Study the drawing (mm; zero at the part's minimum x, y, z) and answer. A direction names the side the tool comes from. Give positions to 0.01 mm unless a question says otherwise; leave off trailing zeros. Write each loop counter-clockwise with the first axis right and the second up, starting at its lowest first coordinate (ties: lowest second). Pieces come first, ordered by that corner, then holes. Notation, with made-up numbers: (-19, 59.25) -> (2, 59.25) arc R28 ccw to (2, 78.25) -> close; hole circle Ø1 at (74, -37). An arc over 180 degrees is marked (long way). Use CSV: the item, a comma, the result in double quotes. Start each with the question number.
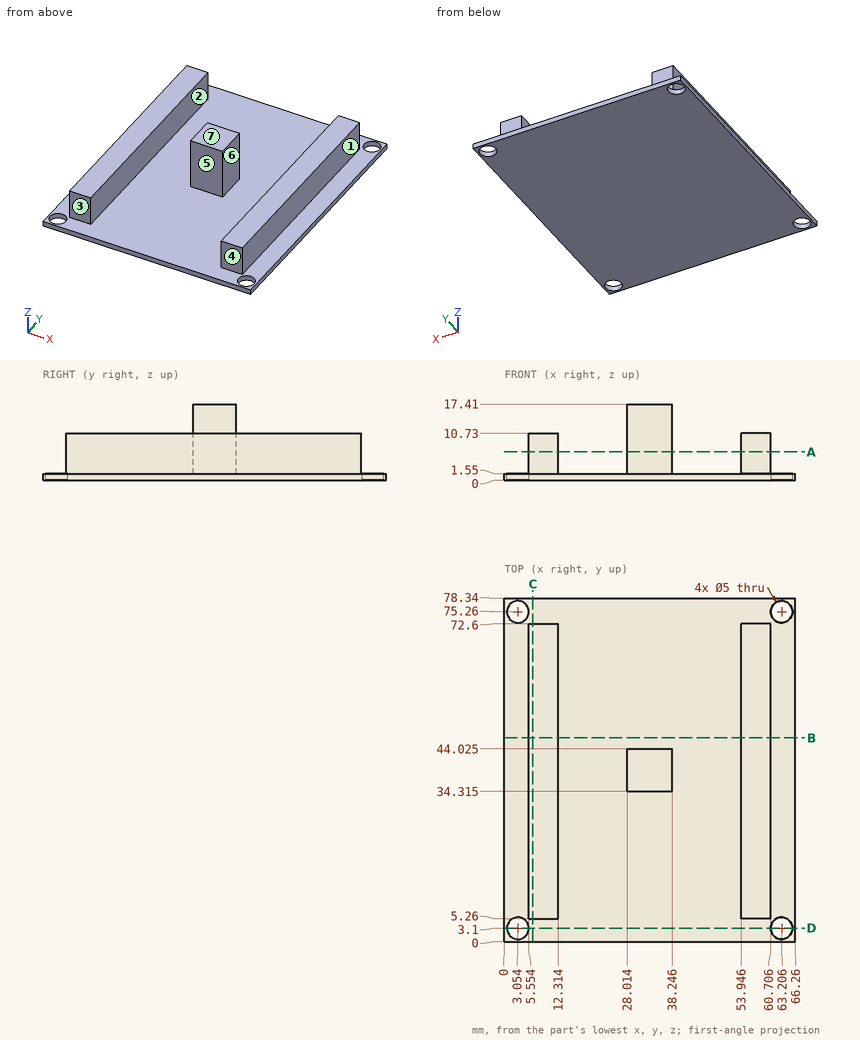
Q1. Straight lines are drawn through the part: L1, parallel to X at y = 41, z = 2; L2, parallel to X at y = 56, z = 5.25; L3, parallel to Z at x = 46.5, y = 47.5. For each, find the intervals that lie inside material, in ascending order.
Q2. Section A-A on z = 6.5 is taken. Give the vertices of the cut face in (x, y) (1 decimal).
Q3. Flat-ended cylindrical pins translate along their axes: pin 1 Ø6.5 at (x, y) = (3.05, 3.1) entering from +Z; pin 2 Ø8 at (y, z) = (40.5, 10.5) entering from +X; pin 3 Ø4.5 at (y, z) = (27.5, 6) entering from -X. Find the tip coordinate at first contact, or state that the pin passes through.
Q4. Section C-C on x = 6.5 is taken. Give the vertices of the cut face in (y, z).
Q5. Section D-D on y = 3.1 is taken. Give the vertices of the cut face in (x, z).
Q6. Section B-B on y = 46.5 is taken. Give the vertices of the cut face in (x, z), then the cut area to 3 significant figures.
Q7. For the marked faces 4, 5, 6 and 7, determine the directions among +Z, -Z, +X, -X, +Y, -Y from which every point of the face is accessible in a straight line to the end or side of a thin tool.
Q8. The mould has two halves that part along X. Classify the marked faces 1, 2 and 3: +X half, -X half, draft (parallel to the pull), parting line (faces both ways), or undercut.
Output:
1,L1,"5.55 to 12.31, 28.01 to 38.25, 53.95 to 60.71"
1,L2,"5.55 to 12.31, 53.95 to 60.71"
1,L3,"0 to 1.55"
2,outline,"(5.6, 5.3) -> (12.3, 5.3) -> (12.3, 72.6) -> (5.6, 72.6) -> close; (28, 34.3) -> (38.2, 34.3) -> (38.2, 44) -> (28, 44) -> close; (53.9, 5.3) -> (60.7, 5.3) -> (60.7, 72.6) -> (53.9, 72.6) -> close"
3,pin 1,"z = 1.55"
3,pin 2,"x = 60.71"
3,pin 3,"x = 5.55"
4,outline,"(0, 0) -> (78.34, 0) -> (78.34, 1.55) -> (72.6, 1.55) -> (72.6, 10.73) -> (5.26, 10.73) -> (5.26, 1.55) -> (0, 1.55) -> close"
5,outline,"(0, 0) -> (0.55, 0) -> (0.55, 1.55) -> (0, 1.55) -> close; (5.55, 0) -> (60.71, 0) -> (60.71, 1.55) -> (5.55, 1.55) -> close; (65.71, 0) -> (66.26, 0) -> (66.26, 1.55) -> (65.71, 1.55) -> close"
6,outline,"(0, 0) -> (66.26, 0) -> (66.26, 1.55) -> (60.71, 1.55) -> (60.71, 10.73) -> (53.95, 10.73) -> (53.95, 1.55) -> (12.31, 1.55) -> (12.31, 10.73) -> (5.55, 10.73) -> (5.55, 1.55) -> (0, 1.55) -> close"
6,area,"227 mm²"
7,face 4,"+Z, +X, -X, -Y"
7,face 5,"+Z, -Y"
7,face 6,"+Z, +Y, -Y"
7,face 7,"+Z, +X, -X, +Y, -Y"
8,face 1,"+X half"
8,face 2,"undercut"
8,face 3,"draft"
